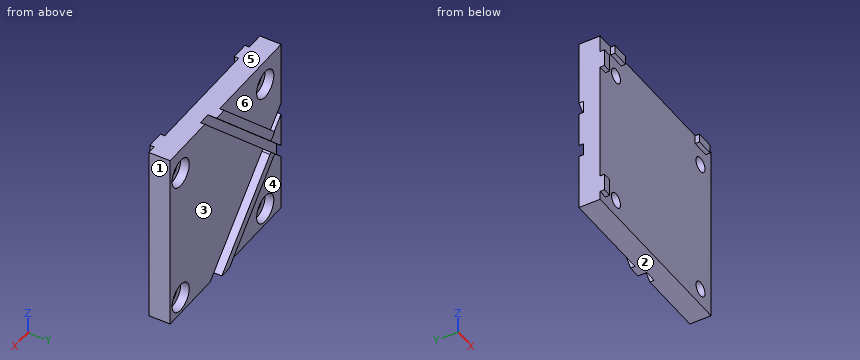
Autodesk Inventor part; units mm, degrees
ref_plane "YZ Plane" through (0, 0, 0) normal (1, 0, 0) x (0, 1, 0)
ref_plane "XZ Plane" through (0, 0, 0) normal (0, 1, 0) x (-1, 0, 0)
ref_plane "XY Plane" through (0, 0, 0) normal (0, 0, 1) x (1, 0, 0)
sketch "Sketch1" plane through (0, 0, 0) normal (0, 1, 0) x (-1, 0, 0)
  line L0 (20, 20) -> (-20, 20)
  line L1 (-20, 20) -> (-20, -20)
  line L2 (-20, -20) -> (20, -20)
  line L3 (20, -20) -> (20, 20)
  line L4 (20, 20) -> (-20, -20) construction
  point P0 (0, 0)
  point P1 (0, 0)
  dimension "d6" = 40
  dimension "d7" = 40
extrude "Extrusion2" add sketch "Sketch1" along normal blind 4.9
sketch "Sketch2" plane through (0, 4.9, 0) normal (0, 1, 0) x (1, 0, 0)
  line L0 (-19.8943, 8.5431) -> (-13.3498, 8.5431) construction
  line L1 (-16.5463, 1.4142) -> (2.0395, 20)
  line L2 (20, 20) -> (-20, 20)
  line L3 (-20, 20) -> (-20, -20)
  line L4 (-20, 0) -> (20, 0)
  line L5 (20, -20) -> (20, 20)
  line L6 (-16.5463, 1.4142) -> (-17.9605, 2.8284)
  line L7 (-17.9605, 2.8284) -> (-0.7889, 20)
  line L8 (-16.5463, -1.4142) -> (2.0395, -20)
  line L9 (20, -20) -> (-20, -20)
  line L10 (-16.5463, -1.4142) -> (-17.9605, -2.8284)
  line L11 (-17.9605, -2.8284) -> (-0.7889, -20)
  line L12 (-16.5463, 1.4142) -> (-12.694, -2.4381) construction
  point P0 (0, 0)
  dimension "d17" = 12.7
  dimension "d18" = 135
  dimension "d19" = 2
  dimension "d51" = 2
extrude "Extrusion3" add sketch "Sketch2" along normal blind 1 contours L6 L7 L2 L1 | L9 L11 L10 L8
sketch "Sketch3" plane through (0, 4.9, 0) normal (0, 1, 0) x (1, 0, 0)
  line L0 (-20, -20) -> (-20, 20) construction
  line L1 (-20, 20) -> (-0.7889, 20) construction
  line L2 (-17.9605, 2.8284) -> (-0.7889, 20) construction
  line L3 (-16.5463, 1.4142) -> (-17.9605, 2.8284) construction
  line L4 (2.0395, 20) -> (-16.5463, 1.4142) construction
  line L5 (2.0395, 20) -> (20, 20) construction
  line L6 (20, 20) -> (20, -20) construction
  line L7 (20, -20) -> (2.0395, -20) construction
  line L8 (2.0395, -20) -> (-0.7889, -20) construction
  line L9 (-0.7889, -20) -> (-20, -20) construction
  line L10 (-0.7889, 20) -> (2.0395, 20) construction
  line L11 (-16.5463, -1.4142) -> (2.0395, -20) construction
  line L12 (-17.9605, -2.8284) -> (-16.5463, -1.4142) construction
  line L13 (-0.7889, -20) -> (-17.9605, -2.8284) construction
  line L14 (2.0395, -20) -> (20, -20)
  line L15 (-20, 20) -> (-20, -20)
  line L16 (20, 20) -> (2.0395, 20)
  line L17 (-17.9605, 2.8284) -> (-16.5463, 1.4142)
  line L18 (2.0395, 20) -> (-16.5463, 1.4142)
  line L19 (-17.9605, 0) -> (-20, -2.0395)
  line L20 (2.0395, -20) -> (-16.5463, -1.4142)
  line L21 (-17.9605, 0) -> (-20, 2.0395)
  line L22 (2.0395, -20) -> (-16.5463, -1.4142)
  line L23 (-16.5463, 1.4142) -> (2.0395, 20)
  line L24 (4.8679, -20) -> (-15.1321, 0)
  line L25 (-16.5463, 1.4142) -> (-20, 4.8679)
  line L26 (-20, -4.8679) -> (-16.5463, -1.4142)
  line L27 (-15.1321, 0) -> (4.8679, 20)
  line L28 (-20, -2.0395) -> (-20, -4.8679)
  line L29 (-20, 2.0395) -> (-20, 4.8679)
extrude "Extrusion4" cut sketch "Sketch3" against normal blind 1 contours L20 L26 L15 L19 L21 L25 L17 L18 L16 L27 L24 L14
sketch "Sketch4" plane through (0, 4.9, 0) normal (0, 1, 0) x (1, 0, 0)
  line L0 (16, -16) -> (-16, -16)
  line L1 (-16, -16) -> (-16, 16)
  line L2 (-16, 16) -> (16, 16)
  line L3 (16, 16) -> (16, -16)
  line L4 (16, -16) -> (-16, 16) construction
  line L5 (-16, -16) -> (16, 16) construction
  point P0 (0, 0)
  dimension "d27" = 32
  dimension "d28" = 32
hole "Hole1" at (-16, 4.9, -16) at (16, 4.9, -16) at (16, 4.9, 16) at (-16, 4.9, 16) direction (0, -1, 0) diameter 3.4 end through all counterbore diameter 6.5 counterbore depth 2
move faces "Move1" translate (-2, 0, 0) faces at (-20, 1.3, -1.6226)
move faces "Move2" translate (0, 0, 2) faces at (0.0132, 1.3, 20)
sketch "Sketch5" plane through (0, 0, 0) normal (0, -1, 0) x (1, 0, 0)
  line L0 (-22, -20) -> (-22, 22) construction
  line L1 (-0.7889, -20) -> (-22, -20)
  line L2 (-22, 22) -> (-20, 22) construction
  line L3 (-20, 20) -> (-20, -20) construction
  line L4 (-20, -20) -> (-22, -20) construction
  line L5 (-22, -20) -> (-22, 22) construction
  line L6 (-22, 22) -> (20, 22) construction
  line L7 (20, 22) -> (20, -20) construction
  line L8 (-22, 22) -> (20, 22) construction
  line L9 (20, 22) -> (20, 20) construction
  line L10 (20, 20) -> (-20, 20) construction
  line L11 (-22, 20) -> (-22, 22) construction
  line L12 (-22, 22) -> (1.2111, 22) construction
  line L13 (-14, 22) -> (-18, 22)
  line L14 (-18, 22) -> (-18, 20)
  line L15 (-18, 20) -> (-14, 20)
  line L16 (-14, 20) -> (-14, 22)
  line L17 (18, 20) -> (14, 20)
  line L18 (14, 20) -> (14, 22)
  line L19 (14, 22) -> (18, 22)
  line L20 (18, 22) -> (18, 20)
  line L21 (0, 0) -> (0, 24.7178)
  line L22 (-20, 14) -> (-22, 14)
  line L23 (-22, 14) -> (-22, 18)
  line L24 (-22, 18) -> (-20, 18)
  line L25 (-20, 18) -> (-20, 14)
  line L26 (-20, -18) -> (-22, -18)
  line L27 (-22, -18) -> (-22, -14)
  line L28 (-22, -14) -> (-20, -14)
  line L29 (-20, -14) -> (-20, -18)
  line L30 (0, 0) -> (-29.8297, 0)
  dimension "d42" = 2
  dimension "d43" = 2
  dimension "d46" = 28
  dimension "d47" = 4
  dimension "d49" = 4
  dimension "d50" = 28
extrude "Extrusion5" add sketch "Sketch5" along normal blind 1
fillet "Fillet2" radius 0.5 3 edges at (-16.5463, 4.9, -1.4142) (-17.9605, 4.4, 0) (-16.5463, 4.9, 1.4142)
equation "\"d6\" = edge"
equation "\"d7\" = edge"
equation "\"d14\" = workingThickness"
equation "\"d19\" = 2 * upstand"
equation "\"d21\" = upstand"
equation "\"d25\" = glueGrooveDepth"
equation "\"d27\" = holePatternEdge"
equation "\"d28\" = d27"
equation "\"d44\" = upstand"
equation "\"edge\" = 40"
equation "\"holePatternEdge\" = 32"
equation "\"workingThickness\" = 4.9"
equation "\"cubeEdge\" = 25.4"
equation "\"upstand\" = 1"
equation "\"glueGrooveDepth\" = 1"
properties part number "FAB-OX0006"
The model under review builds one solid part; all positions refer to its coordinate system, in mm. Face numbers are marked on the shaded views. A direction names the side the tool comes from. Round coordinates to 2 decimals unless told otherwise and drop trailing zeros. Loops run counter-clockwise (first coordinate to the right, second up) from the corner with the lowest first, then second, coordinate; pieces in that order, holes last. Notation, with made-up numbers: (-31, -4) -> (16, -4) arc R14 ccw to (16, 11) -> close; hole circle Ø4 at (30.5, 45). An arc over 180 degrees is marked (long way). Answer as CSV lines item,"result".
1) Add section B-B on z = -15. Write out the cut boundary in (x, y), plus the area to 3 significant figures.
Geometry results:
outline,"(-22, -1) -> (-20, -1) -> (-20, 0) -> (-17.37, 0) -> (-17.37, 2.9) -> (-19.09, 2.9) -> (-19.09, 4.9) -> (-22, 4.9) -> close; (-14.63, 0) -> (14.63, 0) -> (14.63, 2.9) -> (12.91, 2.9) -> (12.91, 4.9) -> (-0.13, 4.9) -> (-0.13, 3.9) -> (-2.96, 3.9) -> (-2.96, 5.9) -> (-5.79, 5.9) -> (-5.79, 4.9) -> (-12.91, 4.9) -> (-12.91, 2.9) -> (-14.63, 2.9) -> close; (17.37, 0) -> (20, 0) -> (20, 4.9) -> (19.09, 4.9) -> (19.09, 2.9) -> (17.37, 2.9) -> close"
area,"167 mm²"
2) Tool access review of the marked faces 4, 5 and 6: name each direction out of +Z, -Z, +X, -X, +Y, -Y from which nothing blocks a thin tool from reaching the whole face with its end or side.
Geometry results:
face 4,"-Z, -X, +Y"
face 5,"+Z, +X, -X, +Y, -Y"
face 6,"+Z, -X, +Y"
3) For P1, Ø0.8, axis at x = -21.5, y = -0.5, coming from the +Z side; P2, Ø5, axis at x = 8, z = -10, coming from the +Y side; P3, Ø0.5, axis at x = 15, y = -0.5, coming from the -Z side, all flat-tipped, find the tip position at first contact; note any pin that passes through.
Geometry results:
P1,"stops at z = 18"
P2,"stops at y = 4.9"
P3,"stops at z = 20"
4) Add section A-A on x = 16. Write out the cut boundary in (y, z), plus the area to 3 significant figures.
Geometry results:
outline,"(-1, 20) -> (0, 20) -> (0, 17.7) -> (2.9, 17.7) -> (2.9, 19.25) -> (4.9, 19.25) -> (4.9, 22) -> (-1, 22) -> close; (0, -20) -> (4.9, -20) -> (4.9, -19.25) -> (2.9, -19.25) -> (2.9, -17.7) -> (0, -17.7) -> close; (0, -14.3) -> (2.9, -14.3) -> (2.9, -12.75) -> (4.9, -12.75) -> (4.9, 12.75) -> (2.9, 12.75) -> (2.9, 14.3) -> (0, 14.3) -> close"
area,"162 mm²"
5) To check wall thickness, follow line 1 along X through (y, z) = (3.8, -16); line 2 along X through (y, z) = (1.3, 16); line 3 along Z through (x, y) = (16, 3.6). State the ranges of each line that lie inside material, in increasing order. Write a range as from..to.
Geometry results:
line 1,"x = -22..-19.25, -12.75..12.75, 19.25..20"
line 2,"x = -22..-17.7, -14.3..14.3, 17.7..20"
line 3,"z = -20..-19.25, -12.75..12.75, 19.25..22"
6) Draft analysis for pull direction Z (two halves, no side actions). For the marked faces 1, 2 and 3, state which applies: pulls with the +Z half, pulls with the -Z half, needs draft (parallel to the pull), parting line crosses it, or undercut.
Geometry results:
face 1,"needs draft"
face 2,"pulls with the -Z half"
face 3,"undercut"
7) Add section D-D on z = 16. Write out the cut boundary in (x, y), plus the area to 3 significant figures.
Geometry results:
outline,"(-22, -1) -> (-20, -1) -> (-20, 0) -> (-17.7, 0) -> (-17.7, 2.9) -> (-19.25, 2.9) -> (-19.25, 4.9) -> (-22, 4.9) -> close; (-14.3, 0) -> (14.3, 0) -> (14.3, 2.9) -> (12.75, 2.9) -> (12.75, 4.9) -> (0.87, 4.9) -> (0.87, 3.9) -> (-1.96, 3.9) -> (-1.96, 5.9) -> (-4.79, 5.9) -> (-4.79, 4.9) -> (-12.75, 4.9) -> (-12.75, 2.9) -> (-14.3, 2.9) -> close; (17.7, 0) -> (20, 0) -> (20, 4.9) -> (19.25, 4.9) -> (19.25, 2.9) -> (17.7, 2.9) -> close"
area,"162 mm²"
8) Add section C-C on x = 9. Write out the cut boundary in (y, z), plus the area to 3 significant figures.
Geometry results:
outline,"(0, -20) -> (4.9, -20) -> (4.9, 22) -> (0, 22) -> close"
area,"206 mm²"
